CAD build for the part. Positions are in the model's coordinates, mm. A direction names the side the tool comes from. Round coordinates to 2 decimals unless told otherwise and drop trailing zeros. Put each result on its own line as item: value. Start each with the question number.
from build123d import *

# Parameters (mm, degrees)
CROQUIS1_W                            = 100
CROQUIS1_H                            = 180
SALIENTE_EXTRUIR1_DEPTH               = 50
TALADRO1_D                            = 12
MATRIZL1_COUNT                        = 5
MATRIZL1_PITCH                        = 20
SIMETR_A1_COPY_1_D                    = 12
SIMETR_A1_COPY_2_D                    = 12
SIMETR_A1_COPY_3_D                    = 12
SIMETR_A1_COPY_4_D                    = 12
TALADRO_DE_MARGEN_PARA_M81_AT_2_COUNT = 2
TALADRO_DE_MARGEN_PARA_M81_AT_2_PITCH = 47.379647221
TALADRO_DE_MARGEN_PARA_M81_AT_3_COUNT = 2
TALADRO_DE_MARGEN_PARA_M81_AT_3_PITCH = 93.023747334
TALADRO_DE_MARGEN_PARA_M81_AT_4_COUNT = 2
TALADRO_DE_MARGEN_PARA_M81_AT_4_PITCH = 23.460534518
TALADRO_DE_MARGEN_PARA_M81_AT_5_COUNT = 2
TALADRO_DE_MARGEN_PARA_M81_AT_5_PITCH = 69.290415903
TALADRO_DE_MARGEN_PARA_M61_D          = 6.6
TALADRO_DE_MARGEN_PARA_M61_DEPTH      = 40
TALADRO_DE_MARGEN_PARA_M61_TIP        = 1.982840043


with BuildPart() as part:
    # Croquis1 → Saliente-Extruir1 (new body)
    with BuildSketch(Plane(origin=(0, 0, 0), x_dir=(1, 0, 0), z_dir=(0, 1, 0))):
        Rectangle(CROQUIS1_W, CROQUIS1_H)
    extrude(amount=SALIENTE_EXTRUIR1_DEPTH)

    # Taladro1 (through all)
    with Locations(Plane(origin=(0, 50, 0), x_dir=(1, 0, 0), z_dir=(0, 1, 0))):
        with Locations((-39.09229064, 77.114510738)):
            taladro1 = Hole(TALADRO1_D / 2)

    # MatrizL1: Taladro1 ×5
    with Locations(*[(i * MATRIZL1_PITCH, 0, 0) for i in range(1, MATRIZL1_COUNT)]):
        add(taladro1, mode=Mode.SUBTRACT)

    # Simetría1: Taladro1 across plane
    add(taladro1.mirror(Plane.XY), mode=Mode.SUBTRACT)

    # Simetría1 copy 1 (through all)
    with Locations(Plane(origin=(20, 50, 0), x_dir=(1, 0, 0), z_dir=(0, 1, 0))):
        with Locations((-39.09229064, -77.114510738)):
            Hole(SIMETR_A1_COPY_1_D / 2)

    # Simetría1 copy 2 (through all)
    with Locations(Plane(origin=(40, 50, 0), x_dir=(1, 0, 0), z_dir=(0, 1, 0))):
        with Locations((-39.09229064, -77.114510738)):
            Hole(SIMETR_A1_COPY_2_D / 2)

    # Simetría1 copy 3 (through all)
    with Locations(Plane(origin=(60, 50, 0), x_dir=(1, 0, 0), z_dir=(0, 1, 0))):
        with Locations((-39.09229064, -77.114510738)):
            Hole(SIMETR_A1_COPY_3_D / 2)

    # Simetría1 copy 4 (through all)
    with Locations(Plane(origin=(80, 50, 0), x_dir=(1, 0, 0), z_dir=(0, 1, 0))):
        with Locations((-39.09229064, -77.114510738)):
            Hole(SIMETR_A1_COPY_4_D / 2)

    # Croquis6 → Taladro de margen para M81 (revolve, cut)
    with BuildSketch(Plane(origin=(-38.819493727, 50, -47.379647221), x_dir=(0, 0, 1), z_dir=(1, 0, 0))):
        Polygon((0, 0), (0, 28.103872786), (4.5, 25.4), (4.5, 0), align=None)
    taladro_de_margen_para_m81 = revolve(axis=Axis((-38.819493727, 56.35, -47.379647221), (0, -1, 0)), mode=Mode.SUBTRACT)

    # Taladro de margen para M81 at 2: Taladro de margen para M81 ×2
    with Locations(*[(0, 0, i * TALADRO_DE_MARGEN_PARA_M81_AT_2_PITCH) for i in range(1, TALADRO_DE_MARGEN_PARA_M81_AT_2_COUNT)]):
        add(taladro_de_margen_para_m81, mode=Mode.SUBTRACT)

    # Taladro de margen para M81 at 3: Taladro de margen para M81 ×2
    with Locations(*[(0, 0, i * TALADRO_DE_MARGEN_PARA_M81_AT_3_PITCH) for i in range(1, TALADRO_DE_MARGEN_PARA_M81_AT_3_COUNT)]):
        add(taladro_de_margen_para_m81, mode=Mode.SUBTRACT)

    # Taladro de margen para M81 at 4: Taladro de margen para M81 ×2
    with Locations(*[(0, 0, i * TALADRO_DE_MARGEN_PARA_M81_AT_4_PITCH) for i in range(1, TALADRO_DE_MARGEN_PARA_M81_AT_4_COUNT)]):
        add(taladro_de_margen_para_m81, mode=Mode.SUBTRACT)

    # Taladro de margen para M81 at 5: Taladro de margen para M81 ×2
    with Locations(*[(0, 0, i * TALADRO_DE_MARGEN_PARA_M81_AT_5_PITCH) for i in range(1, TALADRO_DE_MARGEN_PARA_M81_AT_5_COUNT)]):
        add(taladro_de_margen_para_m81, mode=Mode.SUBTRACT)

    # Simetría2: Taladro de margen para M81 across plane
    add(taladro_de_margen_para_m81.mirror(Plane(origin=(0, 0, 0), x_dir=(0, 0, 1), z_dir=(1, 0, 0))), mode=Mode.SUBTRACT)

    # Simetría2 copy 1 sketch → Simetría2 copy 1 (revolve, cut)
    with BuildSketch(Plane(origin=(38.819493727, 50, 0), x_dir=(0, 0, 1), z_dir=(-1, 0, 0))):
        Polygon((0, 0), (0, -28.103872786), (4.5, -25.4), (4.5, 0), align=None)
    revolve(axis=Axis((38.819493727, 56.35, 0), (0, 1, 0)), mode=Mode.SUBTRACT)

    # Simetría2 copy 2 sketch → Simetría2 copy 2 (revolve, cut)
    with BuildSketch(Plane(origin=(38.819493727, 50, 45.644100113), x_dir=(0, 0, 1), z_dir=(-1, 0, 0))):
        Polygon((0, 0), (0, -28.103872786), (4.5, -25.4), (4.5, 0), align=None)
    revolve(axis=Axis((38.819493727, 56.35, 45.644100113), (0, 1, 0)), mode=Mode.SUBTRACT)

    # Simetría2 copy 3 sketch → Simetría2 copy 3 (revolve, cut)
    with BuildSketch(Plane(origin=(38.819493727, 50, -23.919112702), x_dir=(0, 0, 1), z_dir=(-1, 0, 0))):
        Polygon((0, 0), (0, -28.103872786), (4.5, -25.4), (4.5, 0), align=None)
    revolve(axis=Axis((38.819493727, 56.35, -23.919112702), (0, 1, 0)), mode=Mode.SUBTRACT)

    # Simetría2 copy 4 sketch → Simetría2 copy 4 (revolve, cut)
    with BuildSketch(Plane(origin=(38.819493727, 50, 21.910768682), x_dir=(0, 0, 1), z_dir=(-1, 0, 0))):
        Polygon((0, 0), (0, -28.103872786), (4.5, -25.4), (4.5, 0), align=None)
    revolve(axis=Axis((38.819493727, 56.35, 21.910768682), (0, 1, 0)), mode=Mode.SUBTRACT)

    # Taladro de margen para M61
    with Locations(Plane(origin=(0, 50, 0), x_dir=(1, 0, 0), z_dir=(0, 1, 0))):
        with Locations((0, 52.562788568), (0, 35.649379962), (0, 19.554362094), (0, 0), (0, -18.637205726), (0, -33.368239028), (0, -50.554444547)):
            Hole(TALADRO_DE_MARGEN_PARA_M61_D / 2, depth=TALADRO_DE_MARGEN_PARA_M61_DEPTH)
            with Locations((0, 0, -(TALADRO_DE_MARGEN_PARA_M61_DEPTH + TALADRO_DE_MARGEN_PARA_M61_TIP / 2))):  # 118° drill point
                Cone(0, TALADRO_DE_MARGEN_PARA_M61_D / 2, TALADRO_DE_MARGEN_PARA_M61_TIP, mode=Mode.SUBTRACT)


solid = part.part
(1) Tool access for faces 3 (the flat face through (-1, 0, -1)), 4 (the cylindrical face through (34.427, 37.478, -0.976)): list every direction of +Z, -Z, +X, -X, +Y, -Y with a clear straight run to the whole face (end or side of a thin tool).
(2) Mould opens along Z. For faces 1 (the conical face through (39.478, 22.366, 0.42)), 2 (the flat face through (50, 25, 1)) say: +Z half, -Z half, draft (parallel to the pull), parting line (faces both ways), or undercut.
(3) Cut at A-A on y = 47. Count the separate pieces of the cut face and the enclosed holes in it, and give its area (3 significant figures).
(4) Drill centre lines: line 1 along Z through (x, y) = (24.5, 5); line 2 along Z through (x, y) = (-43.5, 19); line 3 along X through (y, z) = (46.5, 18.5). Where is each one in solid material? Low to high.
(5) Flat gauge pins, fed straight in: pin 1 Ø8 at (x, z) = (-38.82, 0) entering from +Y; pin 2 Ø7 at (x, z) = (20.91, 77.11) entering from +Y. Where does each tip first touch, or does it go through?
Taken from the geometry:
1. face 3: +Z, -Z, +X, -X, -Y
1. face 4: +Y
2. face 1: undercut
2. face 2: draft
3. separate pieces: 1
3. enclosed holes: 27
3. area: 16,000 mm2
4. line 1: -90 to -81.92, -72.31 to 72.31, 81.92 to 90
4. line 2: -90 to -81.19, -73.04 to 73.04, 81.19 to 90
4. line 3: -50 to -41.75, -35.88 to -3.3, 3.3 to 35.88, 41.75 to 50
5. pin 1: y = 24.3
5. pin 2: through
